Study the drawing (mm; zero at the part's minimum x, y, z) and answer. A direction names the side the tool comes from. Coordinates: 2 decimals unless noted, no trailing zeros. Order: outer loops, then holes, each group sorted by start corner. A loop starts at its lowest first (then second) coordinate and runs counter-clockwise, first axis right, second up. Notation, with made-up numbers: M -25.5,22 L -13.5,22 A26 cw -13.5,61 Z; hole C -12,-14.75 d10. An arc over 180 degrees is marked long. Use a Markdown table: item, result. Add a question column.
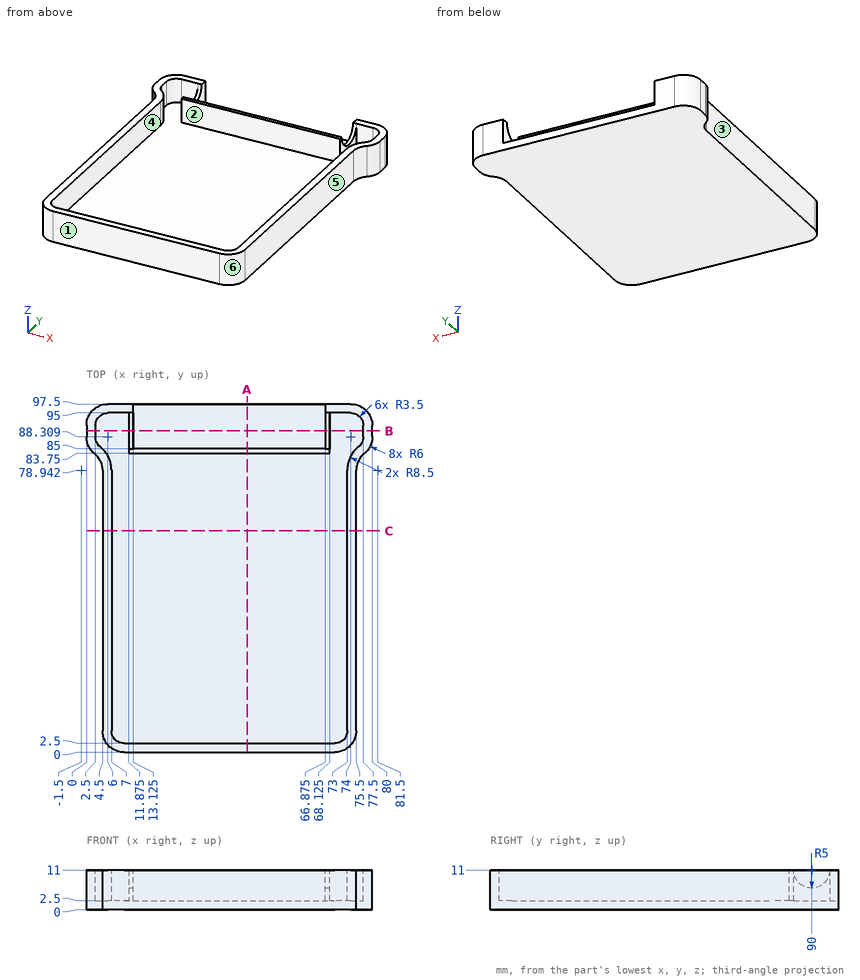
(1) The mould has two halves that part along Y. Classify the marked faces 4, 5 and 6: pulls with the +Y half, pulls with the -Y half, needs draft (parallel to the pull), parting line crosses it, or undercut.
(2) A cutting plane is placed at C-C on y = 62. Write down the section's boundary in (x, z).
(3) Which of the six approach directions +Z, -Z, +X, -X, +Y, -Y give full straight-line access (tool end or side, diameter ignored) to the marked faces 1, 2 and 3?
(4) Straight lines are drawn through the part: line 1 (X direction, y = 90, z = 5.25) (1 decimal); line 2 (Y direction, x = 42, z = 5.5); line 3 (X direction, y = 40, z = 8.75). For each, find the intervals that lie inside material, in ascending order.
(5) A cutting plane is placed at A-A on x = 45. Write down the section's boundary in (y, z).
(6) Given P1, Ø1.5, axis at x = 42.5, y = 76, coming from the -Z side; P2, Ø4, axis at x = 35, y = 93.5, coming from the +Z side; P3, Ø5.5, axis at y = 32.5, z = 6.5, coming from the +X side; P4, Ø2, axis at x = 19, z = 5.5, coming from the +Y side, each flat-ended and moving along its own axis, determine where each tip first touches the part or whether it passes through.
(7) A cutting plane is placed at B-B on y = 90. Write down the section's boundary in (x, z) (1 decimal).
From the geometry:
| question | item | result |
|---|---|---|
| 1 | face 4 | undercut |
| 1 | face 5 | needs draft |
| 1 | face 6 | pulls with the -Y half |
| 2 | outline | M 4.5,0 L 75.5,0 L 75.5,11 L 73,11 L 73,2.5 L 7,2.5 L 7,11 L 4.5,11 Z |
| 3 | face 1 | +Z, -Z, +X, -X, -Y |
| 3 | face 2 | +Z |
| 3 | face 3 | +Z, -Z, -X, -Y |
| 4 | line 1 | x = 0 to 2.5, 11.9 to 13.1, 66.9 to 68.1, 77.5 to 80 |
| 4 | line 2 | y = 0 to 2.5, 83.75 to 85 |
| 4 | line 3 | x = 4.5 to 7, 73 to 75.5 |
| 5 | outline | M 0,0 L 97.5,0 L 97.5,2.5 L 85,2.5 L 85,11 L 83.75,11 L 83.75,2.5 L 2.5,2.5 L 2.5,11 L 0,11 Z |
| 6 | P1 | stops at z = 0 |
| 6 | P2 | stops at z = 2.5 |
| 6 | P3 | stops at x = 75.5 |
| 6 | P4 | stops at y = 85 |
| 7 | outline | M 0,0 L 80,0 L 80,11 L 77.5,11 L 77.5,2.5 L 68.1,2.5 L 68.1,6 L 66.9,6 L 66.9,2.5 L 13.1,2.5 L 13.1,6 L 11.9,6 L 11.9,2.5 L 2.5,2.5 L 2.5,11 L 0,11 Z |
